Autodesk Inventor part; units mm, degrees
ref_plane "Work Plane1" through (14, 0, 0) normal (0, 0, -1) x (1, 0, 0)
ref_plane "YZ Plane" through (0, 0, 0) normal (1, 0, 0) x (0, 1, 0)
ref_plane "XZ Plane" through (0, 0, 0) normal (0, 1, 0) x (-1, 0, 0)
sketch "Sketch1" plane through (0, 0, 0) normal (0, 0, 1) x (1, 0, 0)
  line L0 (0, 2.2) -> (0, 1.3645)
  line L1 (8, 1.5) -> (20, 1.5)
  line L2 (20, 1.5) -> (20, 0)
  line L3 (20, 0) -> (-0.0001, 0)
  line L4 (-4.0001, 0) -> (24, 0)
  line L5 (-0.0001, 0) -> (-0.0001, 2.2)
  line L6 (-0.0001, 2.2) -> (0, 2.2)
  line L7 (8, 1.5) -> (7.6932, 1.3645)
  line L8 (7.6932, 1.3645) -> (0, 1.3645)
  line L9 (0, -0.44) -> (0, 2.64)
  line L10 (7.6932, 1.3645) -> (7.6932, 0) construction
  line L11 (8, 1.5) -> (8, 0) construction
  dimension "d0" = 20
  dimension "d1" = 12
  dimension "d2" = 3
  dimension "d9" = 0.0001
  dimension "d10" = 4.4
  dimension "d13" = 0.3068
  dimension "d14" = 2.729
revolve "Body" add sketch "Sketch1" angle 360 about axis through (20, 0, 0) along (-1, 0, 0)
sketch "Sketch2" plane through (-0.0001, 0, 0) normal (-1, 0, 0) x (0, 0, 1)
  line L0 (0, 3.1754) -> (2.75, 1.5877)
  line L1 (2.75, 1.5877) -> (2.75, -1.5877)
  line L2 (2.75, -1.5877) -> (0, -3.1754)
  line L3 (0, -3.1754) -> (-2.75, -1.5877)
  line L4 (-2.75, -1.5877) -> (-2.75, 1.5877)
  line L5 (-2.75, 1.5877) -> (0, 3.1754)
  point P0 (0, 0)
  point P1 (0, 0)
  dimension "d11" = 5.5
extrude "Head" add sketch "Sketch2" along normal blind 2
sketch "Sketch3" plane through (-2.0001, 0, 0) normal (-1, 0, 0) x (0, 0, 1)
  circle A0 centre (0, 0) radius 2.0625
  point P0 (0, 0)
  dimension "d19" = 4.125
extrude "Indent1" cut sketch "Sketch3" against normal blind 0.4
sketch "Sketch4" plane through (0, 0, 0) normal (0, 0, 1) x (1, 0, 0)
  line L0 (-2.0001, 2.75) -> (-2.0001, 3.1754)
  line L1 (-2.0001, 3.1754) -> (-1.7545, 3.1754)
  line L2 (-1.7545, 3.1754) -> (-2.0001, 2.75)
  line L3 (-2.4001, 0) -> (0.3999, 0)
  line L4 (-0.0001, 3.1754) -> (-2.0001, 3.1754)
  line L5 (-2.0001, 1.5877) -> (-2.0001, 3.1754)
  dimension "d5" = 30
  dimension "d23" = 5.5
revolve "Chamfer1" cut sketch "Sketch4" angle 360 about axis through (-10, 0, 0) along (1, 0, 0)
fillet "Fillet1" radius 0.1 1 edges at (0, -1.3645, 0)
thread "Thread"
chamfer "Chamfer2" distance 0.3067 distance2 0.3068 1 edges at (20, -1.5, 0) measured on face at (20, -0.3888, -0.2119)
ref_plane "Work Plane1" through (14, 0, 0) normal (0, 0, -1) x (1, 0, 0)
equation "\"d0\" = NLG"
equation "\"d1\" = GEL"
equation "\"d2\" = GD"
equation "\"d10\" = SD2"
equation "\"d14\" = BDM"
equation "\"d11\" = SW"
equation "\"d3\" = KOH - SD"
equation "\"d19\" = 0.75 * SW0"
equation "\"d20\" = 0.2 * KOH"
equation "\"d5\" = ANG1"
equation "\"d23\" = SW0"
equation "\"d18\" = RR"
equation "\"d15\" = GEL"
equation "\"d6\" = -0.5 * SPD + 0.5 * GD"
equation "\"NLG\" = 20"
equation "\"GD\" = NND"
equation "\"BDM\" = 2.729"
equation "\"KOH\" = 2"
equation "\"GEL\" = 12"
equation "\"SW\" = 5.5"
equation "\"SW0\" = SW"
equation "\"SPD\" = NND - 1.2269 * PTC"
equation "\"SD2\" = SDH"
equation "\"SD\" = 0"
equation "\"ANG1\" = 30deg"
equation "\"GAL\" = 0.61345 * PTC"
equation "\"GUL\" = 0.61345 * PTC"
equation "\"RR\" = 0.1"
equation "\"WFT\" = 0"
equation "\"GD1\" = THREADDIA - 1.2269 * PTC"
equation "\"THREADDIA\" = 3"
equation "\"SDH\" = 4.4"
equation "\"TOA\" = 30deg"
equation "\"FAWI\" = 90deg"
equation "\"PTC\" = 0.5"
equation "\"NND\" = 3"
equation "\"E0\" = 1.155 * SW"
properties part number "Bolt GB 5784-86-M3 x 20" material "Steel, Mild"
CAD build for the part. Positions are in the model's coordinates, mm. A direction names the side the tool comes from. Coordinates: 2 decimals unless noted, no trailing zeros. Order: outer loops, then holes, each group sorted by start corner. A loop starts at its lowest first (then second) coordinate and runs counter-clockwise, first axis right, second up.
Item 1: Drill centre lines: L1, parallel to X at y = 2.5, z = 0.7; L2, parallel to X at y = -0.5, z = -1.6; L3, parallel to Y at x = -1.8, z = 0. Where is each one in solid material? Low to high.
Check sheet entries:
L1: x = -2 to 0
L2: x = -1.6 to 0
L3: y = -3.1 to -2.06, 2.06 to 3.1
Item 2: Pin check, flat tips, straight feed: pin 1 Ø1.5 at (x, y) = (4, 1) entering from +Z; pin 2 Ø1 at (y, z) = (-0.5, 0) entering from -X. Stop position of each tip, or through.
Check sheet entries:
pin 1: stops at z = 1.34
pin 2: stops at x = -1.6
Item 3: Two-plate mould, pull along X, no slides. Class faces 4 (the face through (-1, 0, -2.75)), 5 (the face through (3.84, 1.3, -0.41)), 6 (the face through (-1.91, 1.46, 2.51)): +X half, -X half, draft (parallel to the pull), parting line (faces both ways), or undercut.
Check sheet entries:
face 4: draft
face 5: undercut
face 6: -X half
Item 4: Band-saw the part on B-B on x = 7.5. List the corners of the cut face in (y, z).
Check sheet entries:
outline: circle Ø2.73 at (0, 0)
Item 5: Band-saw the part on A-A on x = -0.5. List the corners of the cut face in (y, z).
Check sheet entries:
outline: (-3.18, 0) - (-1.59, -2.75) - (1.59, -2.75) - (3.18, 0) - (1.59, 2.75) - (-1.59, 2.75) - close
Item 6: 3-axis set-ups, long thin cutter, end or side, ignore diameter. For faces 1 (the face through (-1.92, 1.44, -2.5)), 2 (the face through (-1.8, -0.8, 1.9)), 3 (the face through (13.93, -1.5, 0.07)): which of +Z, -Z, +X, -X, +Y, -Y reach the whole face in a straight line?
Check sheet entries:
face 1: -Z, -X, +Y
face 2: -X
face 3: +X
